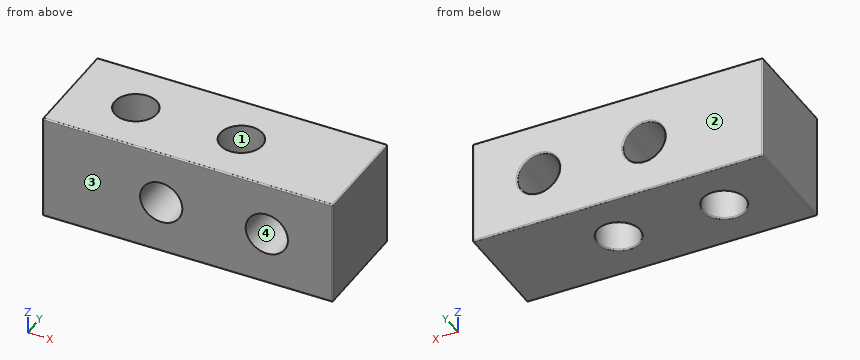
```python
from build123d import *

# Parameters (mm, degrees)
SKETCH_1_W          = 22
SKETCH_1_H          = 8
EXTRUDE_1_DEPTH     = 8
SKETCH_2_R          = 1.6
CUT_EXTRUDE_1_DEPTH = 25.738633754
SKETCH_3_R          = 1.6
CUT_EXTRUDE_2_DEPTH = 25.738633754
FILLET_1_R          = 0.1


with BuildPart() as part:
    # 草图1 → 凸台-拉伸1 (new body)
    with BuildSketch(Plane.XY):
        with Locations((11, -4)):
            Rectangle(SKETCH_1_W, SKETCH_1_H)
    extrude(amount=EXTRUDE_1_DEPTH)

    # 草图2 → 切除-拉伸1 (cut, through all)
    with BuildSketch(Plane.XY.offset(8)):
        with Locations((5, -4)):
            Circle(SKETCH_2_R)
        with Locations((13, -4)):
            Circle(SKETCH_2_R)
    extrude(amount=-CUT_EXTRUDE_1_DEPTH, mode=Mode.SUBTRACT)

    # 草图3 → 切除-拉伸2 (cut, through all)
    with BuildSketch(Plane(origin=(0, 0, 0), x_dir=(1, 0, 0), z_dir=(0, 1, 0))):
        with Locations(Location((17, -4, 0), (0, 0, 270))):
            Circle(SKETCH_3_R)
        with Locations(Location((9, -4, 0), (0, 0, 270))):
            Circle(SKETCH_3_R)
    extrude(amount=-CUT_EXTRUDE_2_DEPTH, mode=Mode.SUBTRACT)

    # 圆角1
    fillet_1_edges = [part.edges().sort_by_distance(p)[0] for p in [
        (22, -4, 8),
        (11, 0, 8),
        (3.4, -4, 0),
        (11.4, -4, 0),
        (17, 0, 2.4),
        (9, 0, 2.4),
        (0, -4, 8),
        (11, 0, 0),
        (22, -4, 0),
        (11, -8, 0),
        (0, -4, 0),
        (0, 0, 4),
        (22, 0, 4),
        (22, -8, 4),
        (0, -8, 4),
        (11, -8, 8),
    ]]
    fillet(fillet_1_edges, radius=FILLET_1_R)


solid = part.part
```
Here's how the part is built. I have some questions about the finished solid (model axes, mm). Face numbers are marked on the shaded views. Give positions to 0.01 mm unless a question says otherwise; leave off trailing zeros. Loops run counter-clockwise (first coordinate to the right, second up) from the corner with the lowest first, then second, coordinate; pieces in that order, holes last. Notation, with made-up numbers: M -10,-0.5 L 12,-0.5 A19 ccw 12,31.5 Z; hole C -28,-36 d2. An arc over 180 degrees is marked long. Return JSON: item names as keys, results as strings.
Item 1: Imagine slicing it at B-B on x = 13. List the corners of the cut face in (y, z) for me, then the cut area to 3 significant figures.
A:
{"outline": "M -8,0.1 A0.1 ccw -7.9,0 L -5.7,0 A0.1 ccw -5.6,0.1 L -5.6,8 L -7.9,8 A0.1 ccw -8,7.9 Z; M -2.4,0.1 A0.1 ccw -2.3,0 L -0.1,0 A0.1 ccw 0,0.1 L 0,7.9 A0.1 ccw -0.1,8 L -2.4,8 Z", "area": "38.4 mm^2"}
Item 2: Imagine slicing it at D-D on z = 7.25. List the corners of the cut face in (x, y) for me.
A:
{"outline": "M 0,-7.9 A0.1 ccw 0.1,-8 L 21.9,-8 A0.1 ccw 22,-7.9 L 22,-0.1 A0.1 ccw 21.9,0 L 0.1,0 A0.1 ccw 0,-0.1 Z; hole C 5,-4 d3.2; hole C 13,-4 d3.2"}
Item 3: Please list where these lines run through material, in increasing order: line 1 (X direction, y = -1, z = 4); line 2 (Y direction, x = 13, z = 2); line 3 (X direction, y = -4.25, z = 4).
A:
{"line 1": "x = 0 to 7.4, 10.6 to 15.4, 18.6 to 22", "line 2": "y = -8 to -5.6, -2.4 to 0", "line 3": "x = 0 to 3.42, 6.58 to 7.4, 10.6 to 11.42, 14.58 to 15.4, 18.6 to 22"}
Item 4: Imagine slicing it at A-A on y = -4. List the corners of the cut face in (x, z) for me, then the cut area to 3 significant figures.
A:
{"outline": "M 0,0.1 A0.1 ccw 0.1,0 L 3.3,0 A0.1 ccw 3.4,0.1 L 3.4,8 L 0.1,8 A0.1 ccw 0,7.9 Z; M 6.6,0.1 A0.1 ccw 6.7,0 L 11.3,0 A0.1 ccw 11.4,0.1 L 11.4,8 L 6.6,8 Z; M 14.6,0.1 A0.1 ccw 14.7,0 L 21.9,0 A0.1 ccw 22,0.1 L 22,7.9 A0.1 ccw 21.9,8 L 14.6,8 Z; hole C 9,4 d3.2; hole C 17,4 d3.2", "area": "109 mm^2"}
Item 5: Thinking about a two-plate mould opening in Y: for the marked faces 1, 2, 3 and 4, which applies, released by +Y, released by -Y, zero draft, split by the parting line, or undercut?
A:
{"face 1": "undercut", "face 2": "released by +Y", "face 3": "released by -Y", "face 4": "zero draft"}
Item 6: Imagine slicing it at C-C on y = -7. List the corners of the cut face in (x, z) for me.
A:
{"outline": "M 0,0.1 A0.1 ccw 0.1,0 L 21.9,0 A0.1 ccw 22,0.1 L 22,7.9 A0.1 ccw 21.9,8 L 0.1,8 A0.1 ccw 0,7.9 Z; hole C 9,4 d3.2; hole C 17,4 d3.2"}
